Build history of the part. All positions in model axes, mm. A direction names the side the tool comes from. Round coordinates to 2 decimals unless told otherwise and drop trailing zeros. Order: outer loops, then holes, each group sorted by start corner. A loop starts at its lowest first (then second) coordinate and runs counter-clockwise, first axis right, second up. Notation, with made-up numbers: (-10.5, -20.75) -> (40.5, -20.75) arc R8 ccw to (40.5, -14.75) -> close; hole circle Ø5 at (-33.75, 33). An arc over 180 degrees is marked (long way). Answer as CSV lines item,"result". Start each with the question number.
```python
from build123d import *

# Parameters (mm, degrees)
SKETCH1_R           = 0.5
BOSS_EXTRUDE1_DEPTH = 0.5
CHAMFER1_SIZE       = 0.08
CHAMFER2_SIZE       = 0.08


with BuildPart() as part:
    # Sketch1 → Boss-Extrude1 (new body, symmetric)
    with BuildSketch(Plane(origin=(0, 0, 0), x_dir=(1, 0, 0), z_dir=(0, 1, 0))):
        with BuildLine():
            Line((-2.5, 0.5), (-3.968626967, 0.5))
            ThreePointArc((-3.968626967, 0.5), (-3.087146594, 2.543526274), (-1.25, 3.799671038))
            Line((-1.25, 3.799671038), (-1.25, 2.5))
            ThreePointArc((-1.25, 2.5), (0, 1.25), (1.25, 2.5))
            Line((1.25, 2.5), (1.25, 3.799671038))
            ThreePointArc((1.25, 3.799671038), (2.919037354, 2.734816434), (3.872983346, 1))
            Line((3.872983346, 1), (2.5, 1))
            ThreePointArc((2.5, 1), (1.5, 0), (2.5, -1))
            Line((2.5, -1), (3.872983346, -1))
            ThreePointArc((3.872983346, -1), (2.736391702, -2.917560702), (0.75, -3.929058411))
            Line((0.75, -3.929058411), (0.75, -2.5))
            ThreePointArc((0.75, -2.5), (0, -1.75), (-0.75, -2.5))
            Line((-0.75, -2.5), (-0.75, -3.929058411))
            ThreePointArc((-0.75, -3.929058411), (-2.916499702, -2.73752251), (-3.968626967, -0.5))
            Line((-3.968626967, -0.5), (-2.5, -0.5))
            ThreePointArc((-2.5, -0.5), (-2, 0), (-2.5, 0.5))
        make_face()
        Circle(SKETCH1_R, mode=Mode.SUBTRACT)
    extrude(amount=BOSS_EXTRUDE1_DEPTH, both=True)

    # Chamfer1
    chamfer1_edges = [part.edges().sort_by_distance(p)[0] for p in [
        (-2, 0.5, 0),
        (-3.234313483, 0.5, 0.5),
        (-2.916499702, 0.5, 2.73752251),
        (-0.75, 0.5, 3.214529206),
        (0, 0.5, 1.75),
        (0.75, 0.5, 3.214529206),
        (2.736391702, 0.5, 2.917560702),
        (-0.5, 0.5, 0),
        (3.186491673, 0.5, 1),
        (1.5, 0.5, 0),
        (3.186491673, 0.5, -1),
        (-3.087146594, 0.5, -2.543526274),
        (2.919037354, 0.5, -2.734816434),
        (1.25, 0.5, -3.149835519),
        (0, 0.5, -1.25),
        (-1.25, 0.5, -3.149835519),
        (-3.234313483, 0.5, -0.5),
    ]]
    chamfer(chamfer1_edges, length=CHAMFER1_SIZE)

    # Chamfer2
    chamfer2_edges = [part.edges().sort_by_distance(p)[0] for p in [
        (-1.25, -0.5, -3.149835519),
        (0, -0.5, -1.25),
        (1.25, -0.5, -3.149835519),
        (2.919037354, -0.5, -2.734816434),
        (3.186491673, -0.5, -1),
        (1.5, -0.5, 0),
        (3.186491673, -0.5, 1),
        (2.736391702, -0.5, 2.917560702),
        (0.75, -0.5, 3.214529206),
        (0, -0.5, 1.75),
        (-0.75, -0.5, 3.214529206),
        (-2.916499702, -0.5, 2.73752251),
        (-3.234313483, -0.5, 0.5),
        (-2, -0.5, 0),
        (-3.234313483, -0.5, -0.5),
        (-3.087146594, -0.5, -2.543526274),
        (-0.5, -0.5, 0),
    ]]
    chamfer(chamfer2_edges, length=CHAMFER2_SIZE)


solid = part.part
```
Q1. Slice it at B-B, the plane y = -0.1. Write the cut outline in (x, z).
Q2. Two-plate mould, pull along Z, no slides. Class faces 1 (the face through (-3.107, 0.006, -2.519)), 2 (the face through (1.25, 0, -3)), 3 (the face through (-3, 0, 0.5)): +Z half, -Z half, draft (parallel to the pull), parting line (faces both ways), or undercut.
Q3. Which spindle directions (+Z, -Z, +X, -X, +Y, -Y) get a long thin tool onto all of the face, cutting with end or side? Do faces 4 (the face through (-3, 0, -0.5)), 5 (the face through (3, 0, 1)), 6 (the face through (-0.75, 0, 3)), 7 (the face through (0, 0.5, 1)). Say none if no direction does.
Q4. Probe L1, parallel to X at y = 0.05, z = 0; L2, parallel to Z at x = 0, y = 0.25; L3, parallel to Z at x = -0.25, y = -0.05. List the from-to ranges inside material, lowest first.
Q5. Slice it at A-A, the plane x = 0. Write the cut outline in (y, z), plus the area to 3 significant figures.
Solutions:
1,outline,"(-3.97, -0.5) arc R4 ccw to (-1.25, -3.8) -> (-1.25, -2.5) arc R1.25 cw to (1.25, -2.5) -> (1.25, -3.8) arc R4 ccw to (3.87, -1) -> (2.5, -1) arc R1 cw to (2.5, 1) -> (3.87, 1) arc R4 ccw to (0.75, 3.93) -> (0.75, 2.5) arc R0.75 cw to (-0.75, 2.5) -> (-0.75, 3.93) arc R4 ccw to (-3.97, 0.5) -> (-2.5, 0.5) arc R0.5 cw to (-2.5, -0.5) -> close; hole circle Ø1 at (0, 0)"
2,face 1,"-Z half"
2,face 2,"draft"
2,face 3,"undercut"
3,face 4,"-X, +Y, -Y"
3,face 5,"+X, +Y, -Y"
3,face 6,"+Z, +Y, -Y"
3,face 7,"+Z, -Z, +X, -X, +Y"
4,L1,"x = -2 to -0.5, 0.5 to 1.5"
4,L2,"z = -1.25 to -0.5, 0.5 to 1.75"
4,L3,"z = -1.28 to -0.43, 0.43 to 1.79"
5,outline,"(-0.5, -1.17) -> (-0.42, -1.25) -> (0.42, -1.25) -> (0.5, -1.17) -> (0.5, -0.58) -> (0.42, -0.5) -> (-0.42, -0.5) -> (-0.5, -0.58) -> close; (-0.5, 0.58) -> (-0.42, 0.5) -> (0.42, 0.5) -> (0.5, 0.58) -> (0.5, 1.67) -> (0.42, 1.75) -> (-0.42, 1.75) -> (-0.5, 1.67) -> close"
5,area,"1.97 mm2"
